Design review of the part built by this model. Coordinates are the model's own, in mm. Give positions to 0.01 mm unless a question says otherwise; leave off trailing zeros. Loops run counter-clockwise (first coordinate to the right, second up) from the corner with the lowest first, then second, coordinate; pieces in that order, holes last. Notation, with made-up numbers: M -5,26.25 L 9,26.25 A9 cw 9,36.25 Z; hole C 70,38 d6. An arc over 180 degrees is marked long. Use CSV: the item, a comma, the result in double quotes.
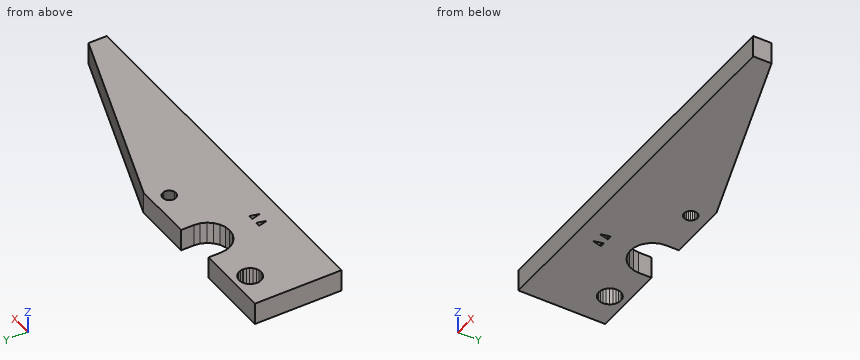
from build123d import *

# Parameters (mm, degrees)
BOSS_EXTRUDE1_DEPTH = 6


with BuildPart() as part:
    # Sketch1 → Boss-Extrude1 (new body)
    with BuildSketch(Plane.XY):
        Polygon((-380.698066711, -270.365836794), (-382.14515244, -269.766434259), (-383.387793127, -268.812922523), (-384.341304863, -267.570281836), (-384.940707398, -266.123196107), (-385.14515244, -264.570281836), (-385.14515244, -261.070281836), (-405.443422321, -261.070281836), (-405.443422321, -284.670281836), (-302.74515244, -284.670281836), (-302.74515244, -279.670281836), (-356.74515244, -261.070281836), (-373.14515244, -261.070281836), (-373.14515244, -264.570281836), (-373.349597482, -266.123196107), (-373.949000017, -267.570281836), (-374.902511753, -268.812922523), (-376.14515244, -269.766434259), (-377.59223817, -270.365836794), (-379.14515244, -270.570281836), align=None)
        Polygon((-359.84515244, -267.129127563), (-360.279278159, -267.308948324), (-360.74515244, -267.370281836), (-361.211026721, -267.308948324), (-361.64515244, -267.129127563), (-362.017944646, -266.843074042), (-362.303998167, -266.470281836), (-362.483818927, -266.036156118), (-362.54515244, -265.570281836), (-362.483818927, -265.104407555), (-362.303998167, -264.670281836), (-362.017944646, -264.29748963), (-361.64515244, -264.01143611), (-361.211026721, -263.831615349), (-360.74515244, -263.770281836), (-360.279278159, -263.831615349), (-359.84515244, -264.01143611), (-359.472360234, -264.29748963), (-359.186306713, -264.670281836), (-359.006485953, -265.104407555), (-358.94515244, -265.570281836), (-359.006485953, -266.036156118), (-359.186306713, -266.470281836), (-359.472360234, -266.843074042), align=None, mode=Mode.SUBTRACT)
        Polygon((-397.620355238, -262.972205625), (-396.896812373, -262.672504357), (-396.120355238, -262.570281836), (-395.343898102, -262.672504357), (-394.620355238, -262.972205625), (-393.999034894, -263.448961493), (-393.522279026, -264.070281836), (-393.222577759, -264.793824701), (-393.14515244, -265.381928384), (-393.14515244, -265.570281836), (-393.247374961, -266.346738972), (-393.547076229, -267.070281836), (-394.023832097, -267.69160218), (-394.64515244, -268.168358048), (-395.368695305, -268.468059315), (-396.14515244, -268.570281836), (-396.921609575, -268.468059315), (-397.64515244, -268.168358048), (-398.266472784, -267.69160218), (-398.743228652, -267.070281836), (-399.042929919, -266.346738972), (-399.14515244, -265.570281836), (-399.018132717, -264.793824701), (-398.718431449, -264.070281836), (-398.241675581, -263.448961493), align=None, mode=Mode.SUBTRACT)
        Polygon((-378.829308223, -275.402326901), (-377.705403878, -279.716351292), (-376.643951896, -275.402326901), (-377.093504107, -277.219304798), (-378.354794122, -277.219304798), align=None, mode=Mode.SUBTRACT)
        Polygon((-381.826259442, -275.402326901), (-380.702355098, -279.716351292), (-379.640903116, -275.402326901), (-380.090455326, -277.219304798), (-381.351745342, -277.219304798), align=None, mode=Mode.SUBTRACT)
    extrude(amount=BOSS_EXTRUDE1_DEPTH)


solid = part.part
(1) Wall thickness on line 1 along Y through (x, z) = (-396, 1.3); line 2 along Y through (x, z) = (-345, 5.5); line 3 along Y through (x, z) = (-361, 3.6): over which ranges is each line inside the solid? List them lowest first. Write a range as [from, to].
A:
line 1,"[-284.67, -268.55], [-262.59, -261.07]"
line 2,"[-284.67, -265.12]"
line 3,"[-284.67, -267.34], [-263.8, -261.07]"
(2) We need section B-B on x = -310.5. State the section outline as (y, z) points, then the cut area to 3 significant figures.
A:
outline,"M -284.67,0 L -277,0 L -277,6 L -284.67,6 Z"
area,"46.0 mm²"
(3) We need section C-C on y = -273.25. State the section outline as (x, z) points.
A:
outline,"M -405.44,0 L -321.38,0 L -321.38,6 L -405.44,6 Z"
(4) Clearance check with flat-ended pins moving along their axes: P1, Ø8, axis at x = -380, y = -265, coming from the -Z side; P2, Ø6, axis at x = -318.5, y = -274, coming from the -Z side. State where each tip first meets the part, or that it passes through.
A:
P1,"through"
P2,"z = 0"
(5) We need section A-A on z = 4.75. Count the separate pieces of the cut face and the enclosed holes in it, then the cut area to 3 significant figures.
A:
separate pieces,"1"
enclosed holes,"4"
area,"1,780 mm²"
